Design review of the part built by this model. Coordinates are the model's own, in mm. A direction names the side the tool comes from. Coordinates: 2 decimals unless noted, no trailing zeros. Order: outer loops, then holes, each group sorted by start corner. A loop starts at its lowest first (then second) coordinate and runs counter-clockwise, first axis right, second up. Notation, with made-up numbers: (24, 25) - (45, 25) arc R15 ccw to (45, 51) - close; hole circle Ø10 at (-25.75, 79). An arc over 180 degrees is marked (long way). Write each question's results on one line, items separated by ' | '. Start each with the question number.
```python
from build123d import *

# Parameters (mm, degrees)
CSK_FOR_M4_COUNTERSUNK_FLAT_HEAD_SCREW1_D           = 4.3
CSK_FOR_M4_COUNTERSUNK_FLAT_HEAD_SCREW1_CSINK_D     = 9.4
CSK_FOR_M4_COUNTERSUNK_FLAT_HEAD_SCREW1_CSINK_ANGLE = 90
PATTERN_CIRCULAR_1_COUNT                            = 6


with BuildPart() as part:
    # Sketch 1 → Revolve 1 (revolve)
    with BuildSketch(Plane.XY):
        with BuildLine():
            Line((0, -5), (60, -5))
            Line((60, -5), (60, 0))
            Line((60, 0), (50, 0))
            ThreePointArc((50, 0), (35.355339059, 35.355339059), (0, 50))
            Line((0, 50), (0, -5))
        make_face()
    revolve(axis=Axis((0, 50, 0), (0, -1, 0)))

    # CSK for M4 Countersunk Flat Head Screw1 (through all)
    with Locations(Plane(origin=(0, 0, -55), x_dir=(1, 0, 0), z_dir=(0, 1, 0))):
        with Locations((0, 0)):
            csk_for_m4_countersunk_flat_head_screw1 = CounterSinkHole(CSK_FOR_M4_COUNTERSUNK_FLAT_HEAD_SCREW1_D / 2, CSK_FOR_M4_COUNTERSUNK_FLAT_HEAD_SCREW1_CSINK_D / 2, counter_sink_angle=CSK_FOR_M4_COUNTERSUNK_FLAT_HEAD_SCREW1_CSINK_ANGLE)

    # Pattern Circular 1: CSK for M4 Countersunk Flat Head Screw1 ×6 about axis
    pattern_circular_1_axis = Axis((0, 0, 0), (0, 1, 0))
    for i in range(1, PATTERN_CIRCULAR_1_COUNT):
        add(csk_for_m4_countersunk_flat_head_screw1.rotate(pattern_circular_1_axis, i * 360 / PATTERN_CIRCULAR_1_COUNT), mode=Mode.SUBTRACT)


solid = part.part
```
(1) Take a section at B-B (z = -27.5). State the section outline as (x, y) points, plus the area to 3 significant figures.
(2) Take a section at D-D (x = 23.5). State the section outline as (y, z) points, plus the area to 3 significant figures.
(3) Tool access review of faces 4 (the face through (46.047, -3.792, -26.047)), 5 (the face through (-23, 0, 45)): name each direction out of +Z, -Z, +X, -X, +Y, -Y from which nothing blocks a thin tool from reaching the whole face with its end or side.
(4) Mouldability with a two-part tool opening along X and no side actions: class faces 1 (the face through (45.36, -2.426, -27.4)), 2 (the face through (-59.94, -2.46, 2.64)), 3 (the face through (1, -5, 1)) as +X half, -X half, draft (parallel to the pull), parting line (faces both ways), or undercut.
(5) Take a section at C-C (z = 55). State the section outline as (x, y) points, plus the area to 3 significant figures.
(6) Clearance check with flat-ended pins moving along their axes: pin 1 (5.5 mm diameter, centred on x = 0, z = 55, fed in from +Y); pin 2 (12 mm diameter, centred on x = -40.5, y = 20, fed in from -Z); pin 3 (3 mm diameter, centred on x = 15, y = 0.5, fed in from +Z). State where each tip first meets the part, or that it passes through.
(7) Take a section at A-A (x = 0). State the section outline as (y, z) points.
(8) To check wall thickness, follow line 1 along X through (y, z) = (-4, 27); line 2 along X through (y, z) = (-4.15, -27.5); line 3 along Z through (x, y) = (13, 20.5). State the ranges of each line that lie inside material, in increasing order. Write a range as [from, to].
Worked out:
1) outline: (-53.33, -5) - (-49.78, -5) - (-49.78, -2.55) - (-52.33, 0) - (-53.33, 0) - close; (-45.48, -5) - (45.48, -5) - (45.48, -2.55) - (42.93, 0) - (41.76, 0) arc R41.76 ccw to (-41.76, 0) - (-42.93, 0) - (-45.48, -2.55) - close; (49.78, -5) - (53.33, -5) - (53.33, 0) - (52.33, 0) - (49.78, -2.55) - close | area: 3,220 mm^2
2) outline: (-5, -55.21) - (0, -55.21) - (0, -44.13) arc R44.13 ccw to (0, 44.13) - (0, 55.21) - (-5, 55.21) - close | area: 3,610 mm^2
3) face 4: +Y, -Y | face 5: +Y
4) face 1: undercut | face 2: parting line | face 3: draft
5) outline: (-23.98, -5) - (-2.15, -5) - (-2.15, -2.55) - (-4.7, 0) - (-23.98, 0) - close; (2.15, -5) - (23.98, -5) - (23.98, 0) - (4.7, 0) - (2.15, -2.55) - close | area: 212 mm^2
6) pin 1: y = -1.95 | pin 2: z = -31.08 | pin 3: z = 58.44
7) outline: (-5, -60) - (0, -60) - (0, -59.7) - (-2.55, -57.15) - (-5, -57.15) - close; (-5, -52.85) - (-2.55, -52.85) - (0, -50.3) - (0, -50) arc R50 ccw to (0, 50) - (0, 50.3) - (-2.55, 52.85) - (-5, 52.85) - close; (-5, 57.15) - (-2.55, 57.15) - (0, 59.7) - (0, 60) - (-5, 60) - close
8) line 1: [-53.58, -49.72], [-45.54, 45.54], [49.72, 53.58] | line 2: [-53.33, -49.78], [-45.48, 45.48], [49.78, 53.33] | line 3: [-43.71, 43.71]
